Could you check a few things on this model? Use its own coordinates, in mm. Face numbers are marked on the shaded views. A direction names the side the tool comes from. Round coordinates to 2 decimals unless told otherwise and drop trailing zeros. Write each question's results on one line, items separated by ' | '. Start each with the question number.
(1) For P1, Ø5, axis at x = 66, y = 11.5, coming from the +Z side; P2, Ø10, axis at x = 41.5, z = -0.5, coming from the -Y side; P3, Ø3, axis at x = 19, y = 14, coming from the +Z side; P4, Ø1.5, axis at x = 51, z = -1.5, coming from the +Y side, each with a flat end and sliding along its axis, tell me the tip position at first contact or that it passes through.
(2) Thinking about a two-plate mould opening in Z: for the marked faces 1, 2 and 3, which applies, +Z half, -Z half, draft (parallel to the pull), parting line (faces both ways), or undercut?
(3) On a 3-axis mill with a long thin cutter (end or side, diameter ignored), from which of +Z, -Z, +X, -X, +Y, -Y can I reach the whole of each face in a straight line? I mean the marked faces 4, 5 and 6. Say none if no direction works.
(4) Imagine slicing it at A-A on z = 14. State how many separate pieces and enclosed holes the cut face has, then the cut area to 3 significant figures.
(5) Please list where these lines run through material, in increasing order: line 1 (Y direction, x = 59, z = 15.5); line 2 (Y direction, x = 67, z = -13); line 3 (Y direction, x = 53, z = 1.5). Write a range as [from, to].
```python
from build123d import *

# Parameters (mm, degrees)
BOSS_EXTRUDE1_DEPTH = 75
SKETCH10_W          = 40
SKETCH10_H          = 5.1


with BuildPart() as part:
    # Sketch1 → Boss-Extrude1 (new body)
    with BuildSketch(Plane(origin=(0, 0, 0), x_dir=(0, 0, -1), z_dir=(1, 0, 0))):
        with BuildLine():
            Line((-18, -42.5), (-5.75, -42.5))
            Line((-5.75, -42.5), (-4.6875, -41.4375))
            Line((-4.6875, -41.4375), (6.604166667, -41.4375))
            Line((6.604166667, -41.4375), (7.666666667, -42.5))
            Line((7.666666667, -42.5), (18, -42.5))
            Line((18, -42.5), (18, -28.152173913))
            Line((18, -28.152173913), (17.5, -28.152173913))
            Line((17.5, -28.152173913), (17.5, -24.5))
            Line((17.5, -24.5), (15.1, -21.666666667))
            Line((15.1, -21.666666667), (18, -18.243055556))
            Line((18, -18.243055556), (18, -11.595935712))
            Line((18, -11.595935712), (15.882352941, -9.072222222))
            Line((15.882352941, -9.072222222), (15.882352941, -7.155555556))
            ThreePointArc((15.882352941, -7.155555556), (15.63583418, -7.424337763), (15.353781513, -7.655555556))
            Line((15.353781513, -7.655555556), (12.382352941, -7.655555556))
            ThreePointArc((12.382352941, -7.655555556), (11.321692769, -7.216215727), (10.882352941, -6.155555556))
            Line((10.882352941, -6.155555556), (10.882352941, -4.955555556))
            ThreePointArc((10.882352941, -4.955555556), (11.321692769, -3.894895384), (12.382352941, -3.455555556))
            Line((12.382352941, -3.455555556), (15.353781513, -3.455555556))
            ThreePointArc((15.353781513, -3.455555556), (15.63583418, -3.686773348), (15.882352941, -3.955555556))
            Line((15.882352941, -3.955555556), (15.882352941, 3.955555556))
            ThreePointArc((15.882352941, 3.955555556), (15.63583418, 3.686773348), (15.353781513, 3.455555556))
            Line((15.353781513, 3.455555556), (12.382352941, 3.455555556))
            ThreePointArc((12.382352941, 3.455555556), (11.321692769, 3.894895384), (10.882352941, 4.955555556))
            Line((10.882352941, 4.955555556), (10.882352941, 6.155555556))
            ThreePointArc((10.882352941, 6.155555556), (11.321692769, 7.216215727), (12.382352941, 7.655555556))
            Line((12.382352941, 7.655555556), (15.353781513, 7.655555556))
            ThreePointArc((15.353781513, 7.655555556), (15.63583418, 7.424337763), (15.882352941, 7.155555556))
            Line((15.882352941, 7.155555556), (15.882352941, 9.072222222))
            Line((15.882352941, 9.072222222), (18, 11.595935712))
            Line((18, 11.595935712), (18, 18.243055556))
            Line((18, 18.243055556), (15.1, 21.666666667))
            Line((15.1, 21.666666667), (17.5, 24.5))
            Line((17.5, 24.5), (17.5, 28.152173913))
            Line((17.5, 28.152173913), (18, 28.152173913))
            Line((18, 28.152173913), (18, 42.5))
            Line((18, 42.5), (7.666666667, 42.5))
            Line((7.666666667, 42.5), (6.604166667, 41.4375))
            Line((6.604166667, 41.4375), (-4.6875, 41.4375))
            Line((-4.6875, 41.4375), (-5.75, 42.5))
            Line((-5.75, 42.5), (-18, 42.5))
            Line((-18, 42.5), (-18, 12))
            Line((-18, 12), (-16.1, 10.1))
            Line((-16.1, 10.1), (-16.1, 5.7))
            ThreePointArc((-16.1, 5.7), (-15.853481239, 5.968782207), (-15.571428571, 6.2))
            Line((-15.571428571, 6.2), (-12.6, 6.2))
            ThreePointArc((-12.6, 6.2), (-11.539339828, 5.760660172), (-11.1, 4.7))
            Line((-11.1, 4.7), (-11.1, 3.3))
            ThreePointArc((-11.1, 3.3), (-11.539339828, 2.239339828), (-12.6, 1.8))
            Line((-12.6, 1.8), (-15.571428571, 1.8))
            ThreePointArc((-15.571428571, 1.8), (-15.853481239, 2.031217793), (-16.1, 2.3))
            Line((-16.1, 2.3), (-16.1, -2.3))
            ThreePointArc((-16.1, -2.3), (-15.853481239, -2.031217793), (-15.571428571, -1.8))
            Line((-15.571428571, -1.8), (-12.6, -1.8))
            ThreePointArc((-12.6, -1.8), (-11.539339828, -2.239339828), (-11.1, -3.3))
            Line((-11.1, -3.3), (-11.1, -4.7))
            ThreePointArc((-11.1, -4.7), (-11.539339828, -5.760660172), (-12.6, -6.2))
            Line((-12.6, -6.2), (-15.571428571, -6.2))
            ThreePointArc((-15.571428571, -6.2), (-15.853481239, -5.968782207), (-16.1, -5.7))
            Line((-16.1, -5.7), (-16.1, -10.1))
            Line((-16.1, -10.1), (-18, -12))
            Line((-18, -12), (-18, -42.5))
        make_face()
    extrude(amount=BOSS_EXTRUDE1_DEPTH)

    # Sketch2 → Cut-Revolve1 (revolve, cut)
    with BuildSketch(Plane.XY, mode=Mode.PRIVATE) as cut_revolve1_sk:
        Polygon((0, 27.5), (0, 33.1), (0.5, 32.6), (74.5, 32.6), (75, 33.1), (75, 27.5), align=None)
    revolve(cut_revolve1_sk.sketch.rotate(Axis((75, 27.5, 0), (-1, 0, 0)), 270), axis=Axis((75, 27.5, 0), (-1, 0, 0)), mode=Mode.SUBTRACT)

    # Sketch3 → Cut-Revolve2 (revolve, cut)
    with BuildSketch(Plane.XY, mode=Mode.PRIVATE) as cut_revolve2_sk:
        Polygon((0, -27.5), (0, -21.9), (0.5, -22.4), (74.5, -22.4), (75, -21.9), (75, -27.5), align=None)
    revolve(cut_revolve2_sk.sketch.rotate(Axis((75, -27.5, 0), (-1, 0, 0)), 270), axis=Axis((75, -27.5, 0), (-1, 0, 0)), mode=Mode.SUBTRACT)

    # Sketch4 → Cut-Revolve3 (revolve, cut)
    with BuildSketch(Plane(origin=(0, 32, 0), x_dir=(-1, 0, 0), z_dir=(0, 1, 0)), mode=Mode.PRIVATE) as cut_revolve3_sk:
        Polygon((-11, -18), (-13.5, -18), (-13.067, -17.567), (-13.067, -10.093383006), (-11, -8.9), align=None)
    revolve(cut_revolve3_sk.sketch.rotate(Axis((11, 32, -8.9), (0, 0, -1)), 180), axis=Axis((11, 32, -8.9), (0, 0, -1)), mode=Mode.SUBTRACT)

    # Sketch5 → Cut-Revolve4 (revolve, cut)
    with BuildSketch(Plane(origin=(0, 32, 0), x_dir=(-1, 0, 0), z_dir=(0, 1, 0)), mode=Mode.PRIVATE) as cut_revolve4_sk:
        Polygon((-61, -18), (-63.5, -18), (-63.067, -17.567), (-63.067, -10.093383006), (-61, -8.9), align=None)
    revolve(cut_revolve4_sk.sketch.rotate(Axis((61, 32, -8.9), (0, 0, -1)), 180), axis=Axis((61, 32, -8.9), (0, 0, -1)), mode=Mode.SUBTRACT)

    # Sketch6 → Cut-Revolve5 (revolve, cut)
    with BuildSketch(Plane(origin=(0, -32, 0), x_dir=(-1, 0, 0), z_dir=(0, 1, 0)), mode=Mode.PRIVATE) as cut_revolve5_sk:
        Polygon((-11, -18), (-13.5, -18), (-13.067, -17.567), (-13.067, -10.093383006), (-11, -8.9), align=None)
    revolve(cut_revolve5_sk.sketch.rotate(Axis((11, -32, -8.9), (0, 0, -1)), 180), axis=Axis((11, -32, -8.9), (0, 0, -1)), mode=Mode.SUBTRACT)

    # Sketch7 → Cut-Revolve6 (revolve, cut)
    with BuildSketch(Plane(origin=(0, -32, 0), x_dir=(-1, 0, 0), z_dir=(0, 1, 0)), mode=Mode.PRIVATE) as cut_revolve6_sk:
        Polygon((-61, -18), (-63.5, -18), (-63.067, -17.567), (-63.067, -10.093383006), (-61, -8.9), align=None)
    revolve(cut_revolve6_sk.sketch.rotate(Axis((61, -32, -8.9), (0, 0, -1)), 180), axis=Axis((61, -32, -8.9), (0, 0, -1)), mode=Mode.SUBTRACT)

    # Sketch8 → Cut-Revolve7 (revolve, cut)
    with BuildSketch(Plane(origin=(0, -24.5, 0), x_dir=(-1, 0, 0), z_dir=(0, 1, 0)), mode=Mode.PRIVATE) as cut_revolve7_sk:
        Polygon((-12, 9.156363636), (-16.131783892, 9.156363636), (-16.389155088, 17.40027692), (-16.988878168, 18), (-12, 18), align=None)
    revolve(cut_revolve7_sk.sketch.rotate(Axis((12, -24.5, 18), (0, 0, -1)), 180), axis=Axis((12, -24.5, 18), (0, 0, -1)), mode=Mode.SUBTRACT)

    # Sketch9 → Cut-Revolve8 (revolve, cut)
    with BuildSketch(Plane(origin=(0, -24.5, 0), x_dir=(-1, 0, 0), z_dir=(0, 1, 0)), mode=Mode.PRIVATE) as cut_revolve8_sk:
        Polygon((-52, 9.156363636), (-56.131783892, 9.156363636), (-56.389155088, 17.40027692), (-56.988878168, 18), (-52, 18), align=None)
    revolve(cut_revolve8_sk.sketch.rotate(Axis((52, -24.5, 18), (0, 0, -1)), 180), axis=Axis((52, -24.5, 18), (0, 0, -1)), mode=Mode.SUBTRACT)

    # Sketch10 → Cut-Revolve9 (revolve, cut)
    with BuildSketch(Plane(origin=(0, 0, 0), x_dir=(-1, 0, 0), z_dir=(0, 1, 0)), mode=Mode.PRIVATE) as cut_revolve9_sk:
        with Locations((-20, -2.55)):
            Rectangle(SKETCH10_W, SKETCH10_H)
    revolve(cut_revolve9_sk.sketch.rotate(Axis((40, 0, 0), (-1, 0, 0)), 180), axis=Axis((40, 0, 0), (-1, 0, 0)), mode=Mode.SUBTRACT)

    # Sketch11 → Cut-Revolve10 (revolve, cut)
    with BuildSketch(Plane(origin=(12, 0, 0), x_dir=(0, 0, -1), z_dir=(1, 0, 0)), mode=Mode.PRIVATE) as cut_revolve10_sk:
        Polygon((-11.5, -33.656363636), (-7.368216108, -33.656363636), (-7.110844912, -41.90027692), (-6.511121832, -42.5), (-11.5, -42.5), align=None)
    revolve(cut_revolve10_sk.sketch.rotate(Axis((12, -42.5, 11.5), (0, 1, 0)), 180), axis=Axis((12, -42.5, 11.5), (0, 1, 0)), mode=Mode.SUBTRACT)

    # Sketch12 → Cut-Revolve11 (revolve, cut)
    with BuildSketch(Plane(origin=(52, 0, 0), x_dir=(0, 0, -1), z_dir=(1, 0, 0)), mode=Mode.PRIVATE) as cut_revolve11_sk:
        Polygon((-11.5, -33.656363636), (-7.368216108, -33.656363636), (-7.110844912, -41.90027692), (-6.511121832, -42.5), (-11.5, -42.5), align=None)
    revolve(cut_revolve11_sk.sketch.rotate(Axis((52, -42.5, 11.5), (0, 1, 0)), 180), axis=Axis((52, -42.5, 11.5), (0, 1, 0)), mode=Mode.SUBTRACT)

    # Sketch13 → Cut-Revolve12 (revolve, cut)
    with BuildSketch(Plane.XY, mode=Mode.PRIVATE) as cut_revolve12_sk:
        Polygon((65.556624327, 0), (67, 2.5), (75, 2.5), (75, 0), align=None)
    revolve(cut_revolve12_sk.sketch.rotate(Axis((75, 0, 0), (-1, 0, 0)), 270), axis=Axis((75, 0, 0), (-1, 0, 0)), mode=Mode.SUBTRACT)

    # Sketch14 → Cut-Revolve13 (revolve, cut)
    with BuildSketch(Plane.XY.offset(-13), mode=Mode.PRIVATE) as cut_revolve13_sk:
        Polygon((58.206616994, 26), (59.4, 28.067), (74.567, 28.067), (75, 28.5), (75, 26), align=None)
    revolve(cut_revolve13_sk.sketch.rotate(Axis((75, 26, -13), (-1, 0, 0)), 270), axis=Axis((75, 26, -13), (-1, 0, 0)), mode=Mode.SUBTRACT)

    # Sketch15 → Cut-Revolve14 (revolve, cut)
    with BuildSketch(Plane.XY.offset(-13), mode=Mode.PRIVATE) as cut_revolve14_sk:
        Polygon((58.206616994, -26), (59.4, -23.933), (74.567, -23.933), (75, -23.5), (75, -26), align=None)
    revolve(cut_revolve14_sk.sketch.rotate(Axis((75, -26, -13), (-1, 0, 0)), 270), axis=Axis((75, -26, -13), (-1, 0, 0)), mode=Mode.SUBTRACT)

    # Sketch16 → Cut-Revolve15 (revolve, cut)
    with BuildSketch(Plane.XY.offset(13), mode=Mode.PRIVATE) as cut_revolve15_sk:
        Polygon((58.206616994, 26), (59.4, 28.067), (74.567, 28.067), (75, 28.5), (75, 26), align=None)
    revolve(cut_revolve15_sk.sketch.rotate(Axis((75, 26, 13), (-1, 0, 0)), 270), axis=Axis((75, 26, 13), (-1, 0, 0)), mode=Mode.SUBTRACT)

    # Sketch17 → Cut-Revolve16 (revolve, cut)
    with BuildSketch(Plane.XY.offset(13), mode=Mode.PRIVATE) as cut_revolve16_sk:
        Polygon((58.206616994, -26), (59.4, -23.933), (74.567, -23.933), (75, -23.5), (75, -26), align=None)
    revolve(cut_revolve16_sk.sketch.rotate(Axis((75, -26, 13), (-1, 0, 0)), 270), axis=Axis((75, -26, 13), (-1, 0, 0)), mode=Mode.SUBTRACT)

    # Sketch18 → Cut-Revolve17 (revolve, cut)
    with BuildSketch(Plane(origin=(19, 0, 0), x_dir=(0, 0, -1), z_dir=(1, 0, 0)), mode=Mode.PRIVATE) as cut_revolve17_sk:
        Polygon((-18, 14), (-18, 18.75), (-12.5, 18.75), (-12.5, 16.6), (5.307179677, 16.6), (5.307179677, 16.4585), (17.4585, 16.4585), (18, 17), (18, 14), align=None)
    revolve(cut_revolve17_sk.sketch.rotate(Axis((19, 14, -18), (0, 0, 1)), 270), axis=Axis((19, 14, -18), (0, 0, 1)), mode=Mode.SUBTRACT)

    # Sketch19 → Cut-Revolve18 (revolve, cut)
    with BuildSketch(Plane(origin=(19, 0, 0), x_dir=(0, 0, -1), z_dir=(1, 0, 0)), mode=Mode.PRIVATE) as cut_revolve18_sk:
        Polygon((-18, -14), (-18, -9.25), (-12.5, -9.25), (-12.5, -11.4), (5.307179677, -11.4), (5.307179677, -11.5415), (17.4585, -11.5415), (18, -11), (18, -14), align=None)
    revolve(cut_revolve18_sk.sketch.rotate(Axis((19, -14, -18), (0, 0, 1)), 270), axis=Axis((19, -14, -18), (0, 0, 1)), mode=Mode.SUBTRACT)

    # Sketch20 → Cut-Revolve19 (revolve, cut)
    with BuildSketch(Plane(origin=(59, 0, 0), x_dir=(0, 0, -1), z_dir=(1, 0, 0)), mode=Mode.PRIVATE) as cut_revolve19_sk:
        Polygon((-18, -14), (-18, -9.25), (-12.5, -9.25), (-12.5, -11.4), (5.307179677, -11.4), (5.307179677, -11.5415), (17.4585, -11.5415), (18, -11), (18, -14), align=None)
    revolve(cut_revolve19_sk.sketch.rotate(Axis((59, -14, -18), (0, 0, 1)), 270), axis=Axis((59, -14, -18), (0, 0, 1)), mode=Mode.SUBTRACT)

    # Sketch21 → Cut-Revolve20 (revolve, cut)
    with BuildSketch(Plane(origin=(59, 0, 0), x_dir=(0, 0, -1), z_dir=(1, 0, 0)), mode=Mode.PRIVATE) as cut_revolve20_sk:
        Polygon((-18, 14), (-18, 18.75), (-12.5, 18.75), (-12.5, 16.6), (5.307179677, 16.6), (5.307179677, 16.4585), (17.4585, 16.4585), (18, 17), (18, 14), align=None)
    revolve(cut_revolve20_sk.sketch.rotate(Axis((59, 14, -18), (0, 0, 1)), 270), axis=Axis((59, 14, -18), (0, 0, 1)), mode=Mode.SUBTRACT)


solid = part.part
```
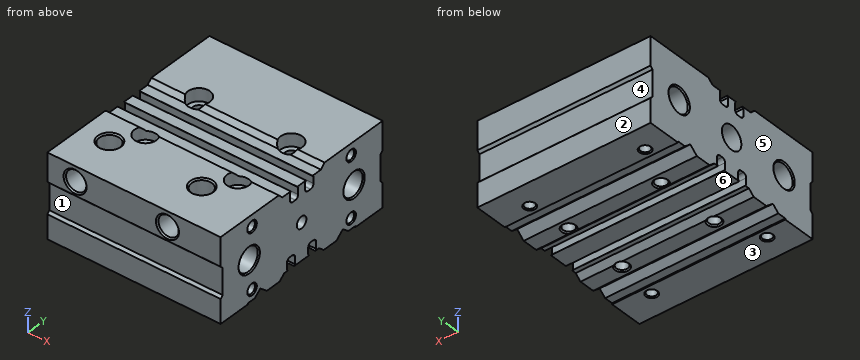
Response:
1) P1: z = 18 | P2: y = -41.44 | P3: through | P4: y = 41.44
2) face 1: undercut | face 2: draft | face 3: -Z half
3) face 4: +X, -X, +Y | face 5: +Z, -Z, -X, +Y, -Y | face 6: -Z, +X, -X
4) separate pieces: 3 | enclosed holes: 6 | area: 5,080 mm²
5) line 1: [-42.5, -18.75], [-9.25, -6.2], [-1.8, 1.8], [6.2, 9.25], [18.75, 42.5] | line 2: [-42.5, -28.07], [-23.93, -7.66], [-3.46, 3.46], [7.66, 23.93], [28.07, 42.5] | line 3: [-41.44, -32.37], [-22.63, 22.63], [32.37, 41.44]
